Can you work these out from the drawing? Everything is in mm from the part's minimum corner. Round coordinates to 2 decimals unless told otherwise and drop trailing zeros. Write each loop counter-clockwise with the first axis right and the second up, starting at its lowest first coordinate (ties: lowest second). Pieces come first, ordered by that corner, then holes. Notation, with made-up numbers: (2, -19) -> (12, -19) arc R24 cw to (12, 3) -> close; hole circle Ø9 at (-29.75, 40.25). An arc over 180 degrees is marked (long way). Answer as CSV lines item,"result". Start each with the question number.
Q1. If we mould it in two halves opening along X, with no side actions, what happens to the marked faces 1, 2 and 3? For each: pulls with the +X half, pulls with the -X half, needs draft (parallel to the pull), parting line crosses it, or undercut.
Q2. Imagine slicing it at A-A on z = 25. Please give me the cut outline in (x, y), and give its area (3 significant figures).
Q3. If I drill on line 1 (Z direction, x = 25, y = 11.5); line 2 (X direction, y = 34.5, z = 48.5), over which ranges is the centre line in solid material (lowest first)? Write a range as [from, to].
Q4. Imagine slicing it at C-C on z = 10.5. Please give me the cut outline in (x, y).
Q5. Imagine slicing it at D-D on x = 15. Please give me the cut outline in (y, z).
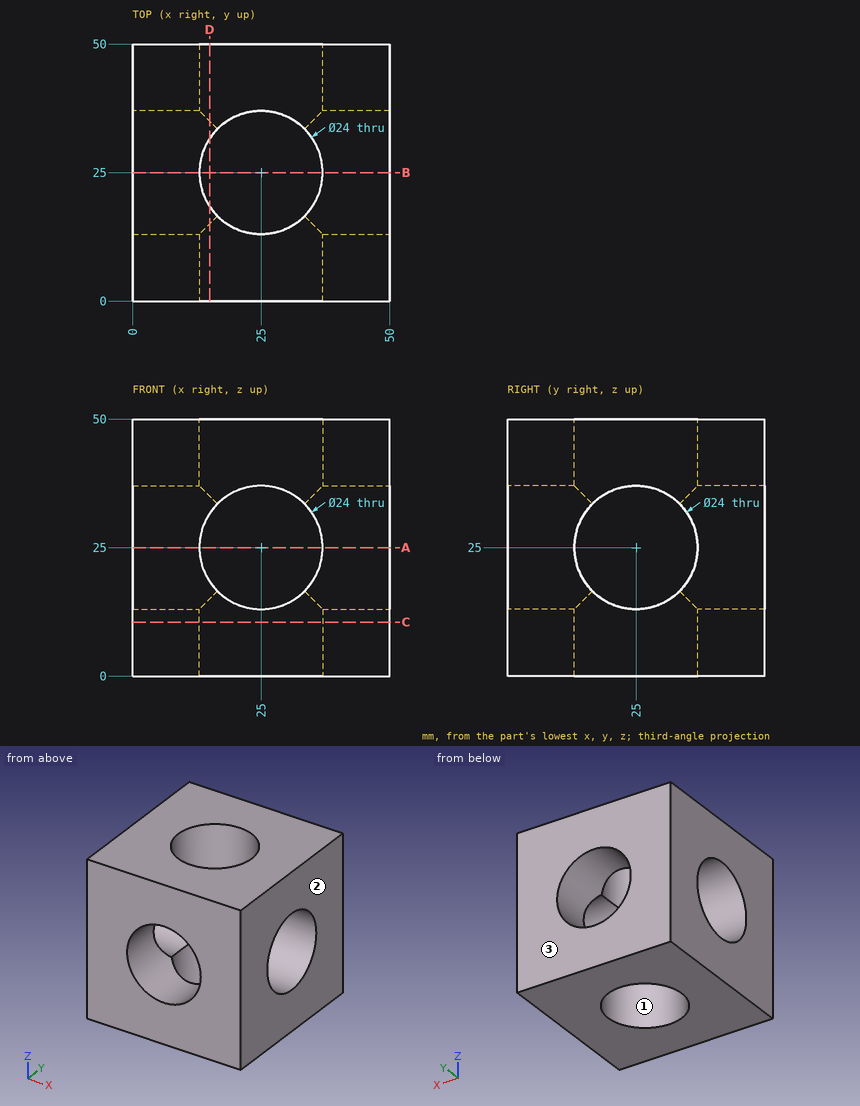
Checks:
1,face 1,"undercut"
1,face 2,"pulls with the +X half"
1,face 3,"needs draft"
2,outline,"(0, 0) -> (13, 0) -> (13, 13) -> (0, 13) -> close; (0, 37) -> (13, 37) -> (13, 50) -> (0, 50) -> close; (37, 0) -> (50, 0) -> (50, 13) -> (37, 13) -> close; (37, 37) -> (50, 37) -> (50, 50) -> (37, 50) -> close"
2,area,"676 mm^2"
3,line 1,"[0, 13], [37, 50]"
3,line 2,"[0, 17.67], [32.33, 50]"
4,outline,"(0, 0) -> (50, 0) -> (50, 50) -> (0, 50) -> close; hole circle Ø24 at (25, 25)"
5,outline,"(0, 0) -> (18.37, 0) -> (18.37, 15) arc R12 cw to (15, 18.37) -> (0, 18.37) -> close; (0, 31.63) -> (15, 31.63) arc R12 cw to (18.37, 35) -> (18.37, 50) -> (0, 50) -> close; (31.63, 0) -> (50, 0) -> (50, 18.37) -> (35, 18.37) arc R12 cw to (31.63, 15) -> close; (31.63, 35) arc R12 cw to (35, 31.63) -> (50, 31.63) -> (50, 50) -> (31.63, 50) -> close"
